```python
from build123d import *

# Parameters (mm, degrees)
SKETCH1_R                                     = 48.312804733
BOSS_EXTRUDE1_DEPTH                           = 24
CBORE_FOR_1_4_SOCKET_HEAD_CAP_SCREW2_AT_COUNT = 2
CBORE_FOR_1_4_SOCKET_HEAD_CAP_SCREW2_AT_PITCH = 61.636013361
CBORE_FOR_1_4_SOCKET_HEAD_CAP_SCREW2_2_COUNT  = 2
CBORE_FOR_1_4_SOCKET_HEAD_CAP_SCREW2_2_PITCH  = 87.166486026
CBORE_FOR_1_4_SOCKET_HEAD_CAP_SCREW2_3_COUNT  = 2
CBORE_FOR_1_4_SOCKET_HEAD_CAP_SCREW2_3_PITCH  = 61.636013361
CIRPATTERN1_COUNT                             = 8


with BuildPart() as part:
    # Sketch1 → Boss-Extrude1 (new body)
    with BuildSketch(Plane(origin=(0, 0, 0), x_dir=(1, 0, 0), z_dir=(0, 1, 0))):
        with Locations(Location((0, 0, 0), (0, 0, 270))):
            Circle(SKETCH1_R)
    extrude(amount=BOSS_EXTRUDE1_DEPTH)

    # Sketch8 → CBORE for 1/4 Socket Head Cap Screw2 (revolve, cut)
    with BuildSketch(Plane(origin=(0, 24, -43.583243013), x_dir=(0, 0, 1), z_dir=(1, 0, 0))):
        Polygon((0, 0), (0, 24), (3.3782, 24), (3.3782, 6.35), (5.55625, 6.35), (5.55625, 0.635), (6.19125, 0), align=None)
    cbore_for_1_4_socket_head_cap_screw2 = revolve(axis=Axis((0, 30.35, -43.583243013), (0, -1, 0)), mode=Mode.SUBTRACT)

    # CBORE for 1/4 Socket Head Cap Screw2 at: CBORE for 1/4 Socket Head Cap Screw2 ×2
    with Locations(*[Vector(-0.7071067811865476, 0, 0.7071067811865476) * (i * CBORE_FOR_1_4_SOCKET_HEAD_CAP_SCREW2_AT_PITCH) for i in range(1, CBORE_FOR_1_4_SOCKET_HEAD_CAP_SCREW2_AT_COUNT)]):
        add(cbore_for_1_4_socket_head_cap_screw2, mode=Mode.SUBTRACT)

    # CBORE for 1_4 Socket Head Cap Screw2 2: CBORE for 1/4 Socket Head Cap Screw2 ×2
    with Locations(*[(0, 0, i * CBORE_FOR_1_4_SOCKET_HEAD_CAP_SCREW2_2_PITCH) for i in range(1, CBORE_FOR_1_4_SOCKET_HEAD_CAP_SCREW2_2_COUNT)]):
        add(cbore_for_1_4_socket_head_cap_screw2, mode=Mode.SUBTRACT)

    # CBORE for 1_4 Socket Head Cap Screw2 3: CBORE for 1/4 Socket Head Cap Screw2 ×2
    with Locations(*[Vector(0.7071067811865476, 0, 0.7071067811865476) * (i * CBORE_FOR_1_4_SOCKET_HEAD_CAP_SCREW2_3_PITCH) for i in range(1, CBORE_FOR_1_4_SOCKET_HEAD_CAP_SCREW2_3_COUNT)]):
        add(cbore_for_1_4_socket_head_cap_screw2, mode=Mode.SUBTRACT)

    # Sketch10 → CBORE for 1/4 Socket Head Cap Screw3 (revolve, cut)
    with BuildSketch(Plane(origin=(30, 24, 0), x_dir=(0, 0, 1), z_dir=(1, 0, 0))):
        Polygon((0, 0), (0, 24), (3.3782, 24), (3.3782, 6.35), (5.55625, 6.35), (5.55625, 0.635), (6.19125, 0), align=None)
    cbore_for_1_4_socket_head_cap_screw3 = revolve(axis=Axis((30, 30.35, 0), (0, -1, 0)), mode=Mode.SUBTRACT)

    # CirPattern1: CBORE for 1/4 Socket Head Cap Screw3 ×8 about axis
    cirpattern1_axis = Axis((0, 0, 0), (0, 1, 0))
    for i in range(1, CIRPATTERN1_COUNT):
        add(cbore_for_1_4_socket_head_cap_screw3.rotate(cirpattern1_axis, i * 360 / CIRPATTERN1_COUNT), mode=Mode.SUBTRACT)


solid = part.part
```
CAD build for the part. Positions are in the model's coordinates, mm. A direction names the side the tool comes from. Coordinates: 2 decimals unless noted, no trailing zeros. Write each loop counter-clockwise with the first axis right and the second up, starting at its lowest first coordinate (ties: lowest second). Pieces come first, ordered by that corner, then holes.
(1) Drill centre lines: probe 1 along X at (y, z) = (20.4, 0); probe 2 along Z at (x, y) = (-20.5, 6.5); probe 3 along X at (y, z) = (7, 19). Where is each one in solid material? Low to high.
(2) 3-axis set-ups, long thin cutter, end or side, ignore diameter. For faces 1 (the face through (-1.015, 8.949, 46.805)), 2 (the face through (25, 17.65, 21)): which of +Z, -Z, +X, -X, +Y, -Y reach the whole face in a straight line?
(3) Two-plate mould, pull along Z, no slides. Class faces 3 (the face through (14.512, 11.832, 46.082)), 4 (the face through (-40.96, 17.65, -2.39)): +Z half, -Z half, draft (parallel to the pull), parting line (faces both ways), or undercut.
(4) Cut at B-B, the plane z = 30. List the corners of the cut face in (x, y) (3 decimals), and give its area (3 significant figures).
(5) Cut at A-A, the plane y = 22.25. Count the separate pieces of the cut face and the enclosed holes in it, and give its area (3 significant figures).
(6) Flat gauge pins, fed straight in: pin 1 (11.5 mm diameter, centred on x = -1.5, z = -44.5, fed in from +Y); pin 2 (10 mm diameter, centred on y = 10.5, z = -24, fed in from -X); pin 3 (3.5 mm diameter, centred on x = 31, z = -2, fed in from +Y); pin 4 (5.5 mm diameter, centred on x = 2.5, z = -32, fed in from +Y). Where does each tip first touch, or does it go through?
(7) Cut at C-C, the plane x = 30. List the corners of the cut face in (y, z) (3 decimals), and give its area (3 significant figures).
Geometry says:
1. probe 1: x = -38.03 to -35.56, -24.44 to 24.44, 35.56 to 38.03
1. probe 2: z = -43.75 to -24.52, -17.91 to 17.91, 24.52 to 43.75
1. probe 3: x = -44.42 to -23.77, -18.66 to 18.66, 23.77 to 44.42
2. face 1: +Y, -Y
2. face 2: +Y
3. face 3: parting line
3. face 4: undercut
4. outline: (-37.87, 0) - (-3.378, 0) - (-3.378, 17.65) - (-5.556, 17.65) - (-5.556, 23.365) - (-6.191, 24) - (-37.87, 24) - close; (3.378, 0) - (37.87, 0) - (37.87, 24) - (6.191, 24) - (5.556, 23.365) - (5.556, 17.65) - (3.378, 17.65) - close
4. area: 1,630 mm2
5. separate pieces: 1
5. enclosed holes: 8
5. area: 6,180 mm2
6. pin 1: stops at y = 24
6. pin 2: stops at x = -44.42
6. pin 3: stops at y = 17.65
6. pin 4: stops at y = 23.76
7. outline: (0, -37.87) - (24, -37.87) - (24, -6.191) - (23.365, -5.556) - (17.65, -5.556) - (17.65, -3.378) - (0, -3.378) - close; (0, 3.378) - (17.65, 3.378) - (17.65, 5.556) - (23.365, 5.556) - (24, 6.191) - (24, 37.87) - (0, 37.87) - close
7. area: 1,630 mm2
